Input: part model. Units: mm. Frame: model coordinates. Face numbers are marked on the shaded views. A direction names the side the tool comes from. Give positions to 0.01 mm unless a question says otherwise; leave off trailing zeros. Loops run counter-clockwise (first coordinate to the right, second up) from the corner with the lowest first, then second, coordinate; pieces in that order, holes last. Notation, with made-up numbers: M 78.25,33 L 125.25,33 A22 cw 125.25,39 Z; hole C 54.25,62 d3. An arc over 180 degrees is marked long. Use CSV: the item, a comma, the result in double quotes. Start each with the question number.
Q1. Section B-B, the plane x = 20. Output: boundary loops of the cut face in (y, z), plus the area to 3 significant figures.
Q2. Section C-C, the plane z = 94.5. Output: boundary loops of the cut face in (x, y).
Q3. Pull-direction query (Y, two-part tool) for the marked faces 4, 5, 6 and 7; classes: released by +Y, released by -Y, zero draft, split by the parting line, or undercut.
Q4. Pin query (flat end, axial travel): pin 1 (10 mm diameter, centred on x = 40.5, y = 33.5, fed in from -Z); pin 2 (21 mm diameter, centred on x = 8, y = -30, fed in from -Z); pin 3 (8 mm diameter, centred on y = 12, z = 49, fed in from +X). Return the tip coordinate at first contact, or that it passes through.
Q5. Material intervals for line 1 along Y through (x, z) = (90, 5.25); line 2 along Y through (x, z) = (32.5, 84.5); line 3 along Z through (x, y) = (18, 29), sorted ascending.
Q6. Section D-D, the plane y = 57. Output: boundary loops of the cut face in (x, z).
Q7. Reachability of the marked faces 1, 2 and 3 from +Z, -Z, +X, -X, +Y, -Y: full face, straight path, thin tool, end or side. Return the list, or none.
Q8. Section A-A, the plane x = 93.5. Output: boundary loops of the cut face in (y, z).
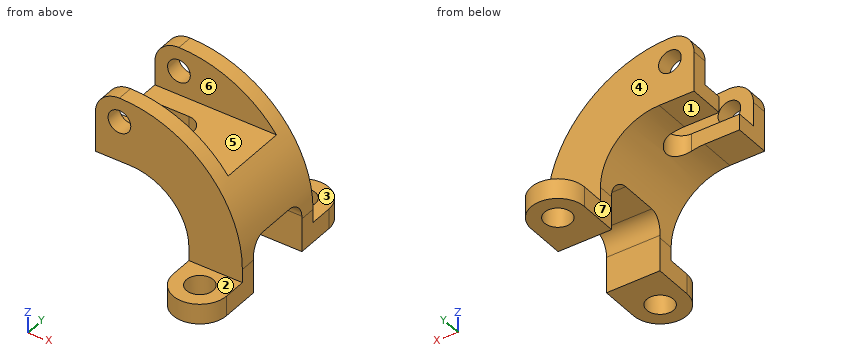
from build123d import *

# Parameters (mm, degrees)
SKETCH_R          = 8.5
PAD_DEPTH         = 38
SKETCH001_W       = 52
SKETCH001_H       = 36
POCKET_DEPTH      = 0.001
POCKET_DEPTH_BACK = 110.001
POCKET001_DEPTH   = 81.001
SKETCH003_R       = 10
PAD001_DEPTH      = 15


with BuildPart() as part:
    # Sketch (on XZ_Plane of Origin) → Pad (new body, symmetric)
    with BuildSketch(Plane.XZ):
        with BuildLine():
            Line((70, 0), (110, 0))
            Line((110, 0), (110, 25))
            ThreePointArc((110, 25), (83.053824, 90.053824), (18, 117))
            ThreePointArc((18, 117), (5.272078, 111.727922), (0, 99))
            Line((0, 99), (0, 69))
            Line((0, 69), (26, 69))
            ThreePointArc((70, 25), (57.112698, 56.112698), (26, 69))
            Line((70, 25), (70, 0))
        make_face()
        with Locations((18, 99)):
            Circle(SKETCH_R, mode=Mode.SUBTRACT)
    extrude(amount=PAD_DEPTH, both=True)

    # Sketch001 (on YZ_Plane of Origin) → Pocket (cut, two sides)
    with BuildSketch(Plane.YZ) as pocket_sk:
        with BuildLine():
            Line((-26, 0), (-26, 27))
            ThreePointArc((-14, 39), (-22.485281, 35.485281), (-26, 27))
            Line((-14, 39), (14, 39))
            ThreePointArc((26, 27), (22.485281, 35.485281), (14, 39))
            Line((26, 27), (26, 0))
            Line((26, 0), (-26, 0))
        make_face()
        with Locations((0, 99)):
            Rectangle(SKETCH001_W, SKETCH001_H)
    extrude(amount=-POCKET_DEPTH, mode=Mode.SUBTRACT)
    extrude(pocket_sk.sketch, amount=POCKET_DEPTH_BACK, mode=Mode.SUBTRACT)

    # Sketch002 (on Face14 of Pocket) → Pocket001 (cut, through all)
    with BuildSketch(Plane.XY.offset(81)):
        with BuildLine():
            ThreePointArc((0, 11), (-11, 0), (0, -11))
            Line((0, -11), (36, -11))
            ThreePointArc((36, -11), (47, 0), (36, 11))
            Line((0, 11), (36, 11))
        make_face()
    extrude(amount=-POCKET001_DEPTH, mode=Mode.SUBTRACT)

    # Sketch003 (on XY_Plane of Origin) → Pad001 (join)
    with BuildSketch(Plane.XY):
        with BuildLine():
            Line((70, 38), (70, 55))
            ThreePointArc((70, 55), (90, 75), (110, 55))
            Line((110, 55), (110, 38))
            Line((110, 38), (70, 38))
        make_face()
        with Locations((90, 55)):
            Circle(SKETCH003_R, mode=Mode.SUBTRACT)
    pad001 = extrude(amount=PAD001_DEPTH)

    # Mirrored: Pad001 across XZ
    add(pad001.mirror(Plane.XZ))


solid = part.part
A:
1,outline,"M -38,69 L -11,69 L -11,81 L -26,81 L -26,90.74 L -38,90.74 Z; M -38,107.26 L -26,107.26 L -26,116.98 L -38,116.98 Z; M 11,69 L 38,69 L 38,90.74 L 26,90.74 L 26,81 L 11,81 Z; M 26,107.26 L 38,107.26 L 38,116.98 L 26,116.98 Z"
1,area,"1,110 mm^2"
2,outline,"M 0,-38 L 10.79,-38 L 10.79,-26 L 0,-26 Z; M 0,26 L 10.79,26 L 10.79,38 L 0,38 Z; M 25.21,-38 L 78.28,-38 L 78.28,-26 L 25.21,-26 Z; M 25.21,26 L 78.28,26 L 78.28,38 L 25.21,38 Z"
3,face 4,"released by +Y"
3,face 5,"undercut"
3,face 6,"undercut"
3,face 7,"zero draft"
4,pin 1,"z = 64.44"
4,pin 2,"z = 69"
4,pin 3,"x = 107.8"
5,line 1,"-75 to -65, -45 to -26, 26 to 45, 65 to 75"
5,line 2,"-38 to -26, 26 to 38"
5,line 3,"69 to 90.5, 107.5 to 117"
6,outline,"M 70.1,0 L 80.2,0 L 80.2,15 L 70.1,15 Z; M 99.8,0 L 109.9,0 L 109.9,15 L 99.8,15 Z"
7,face 1,"-Z, -X, +Y, -Y"
7,face 2,"+Z, +X, -X, -Y"
7,face 3,"+Z, +X, -X, +Y"
8,outline,"M -74.69,0 L -64.37,0 L -64.37,15 L -74.69,15 Z; M -45.63,0 L -26,0 L -26,27 A12 cw -14,39 L 14,39 A12 cw 26,27 L 26,0 L 45.63,0 L 45.63,15 L 38,15 L 38,77.57 L -38,77.57 L -38,15 L -45.63,15 Z; M 64.37,0 L 74.69,0 L 74.69,15 L 64.37,15 Z"
